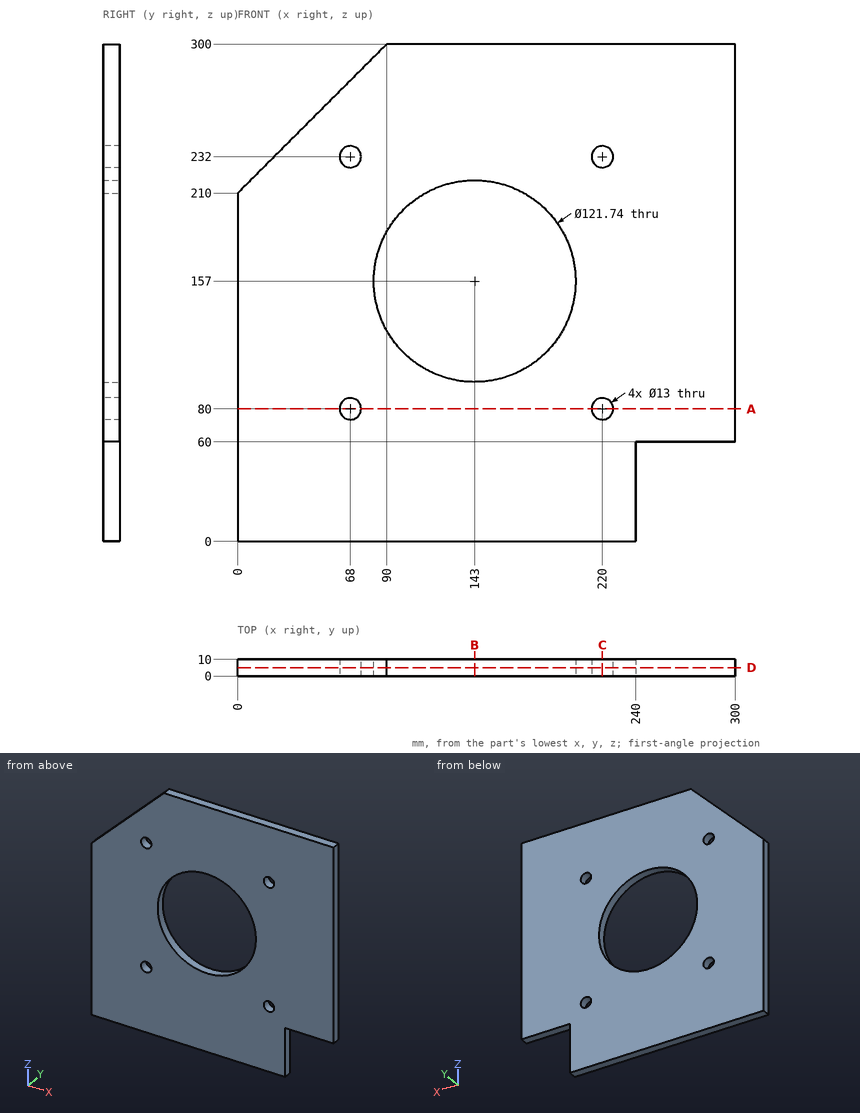
Source: three-view drawing plus pictorial views. Frame: mm from the lowest corner of the part. Give positions to 0.01 mm unless a question says otherwise; leave off trailing zeros. Write each loop counter-clockwise with the first axis right and the second up, starting at its lowest first coordinate (ties: lowest second). Pieces come first, ordered by that corner, then holes. Notation, with made-up numbers: (-4.5, -15) - (1.5, -15) arc R24 cw to (1.5, 19) - close; hole circle Ø6 at (60, 4). An arc over 180 degrees is marked (long way). Write item = value, one per line. Start each with the question number.
1. Section query A-A, the plane z = 80. Output: boundary loops of the cut face in (x, y), then the cut area to 3 significant figures.
2. Section query C-C, the plane x = 220. Output: boundary loops of the cut face in (y, z).
3. Section query D-D, the plane y = 5. Output: boundary loops of the cut face in (x, z), then the cut area to 3 significant figures.
4. First-contact query: pin 1 Ø8 at (x, z) = (68, 232) entering from -Y; pin 2 Ø17 at (x, z) = (68, 80) entering from +Y; pin 3 Ø5 at (y, z) = (4, 19) entering from +X. Flat tips, straight axial feed; report the tip coordinate or a pass-through.
5. Section query B-B, the plane x = 143. Output: boundary loops of the cut face in (y, z), then the cut area to 3 significant figures.
6. Ray query, L1, parallel to Z at x = 68, y = 7.75; L2, parallel to Z at x = 143, y = 3; L3, parallel to Z at x = 244.5, y = 9.5. Return the intervals inside material, ascending.
Check sheet entries:
q1.outline = (0, 0) - (61.5, 0) - (61.5, 10) - (0, 10) - close; (74.5, 0) - (213.5, 0) - (213.5, 10) - (74.5, 10) - close; (226.5, 0) - (300, 0) - (300, 10) - (226.5, 10) - close
q1.area = 2,740 mm2
q2.outline = (0, 0) - (10, 0) - (10, 73.5) - (0, 73.5) - close; (0, 86.5) - (10, 86.5) - (10, 225.5) - (0, 225.5) - close; (0, 238.5) - (10, 238.5) - (10, 300) - (0, 300) - close
q3.outline = (0, 0) - (240, 0) - (240, 60) - (300, 60) - (300, 300) - (90, 300) - (0, 210) - close; hole circle Ø13 at (68, 80); hole circle Ø13 at (68, 232); hole circle Ø121.74 at (143, 157); hole circle Ø13 at (220, 80); hole circle Ø13 at (220, 232)
q3.area = 70,200 mm2
q4.pin_1 = through
q4.pin_2 = 10
q4.pin_3 = 240
q5.outline = (0, 0) - (10, 0) - (10, 96.13) - (0, 96.13) - close; (0, 217.87) - (10, 217.87) - (10, 300) - (0, 300) - close
q5.area = 1,780 mm2
q6.L1 = 0 to 73.5, 86.5 to 225.5, 238.5 to 278
q6.L2 = 0 to 96.13, 217.87 to 300
q6.L3 = 60 to 300
